The model under review builds one solid part; all positions refer to its coordinate system, in mm. Face numbers are marked on the shaded views. A direction names the side the tool comes from. Give positions to 0.01 mm unless a question says otherwise; leave off trailing zeros. Order: outer loops, then holes, each group sorted by start corner. A loop starts at its lowest first (then second) coordinate and runs counter-clockwise, first axis right, second up. Notation, with made-up numbers: (38.25, -13.5) - (73.25, -13.5) arc R15 ccw to (73.25, 10.5) - close; hole circle Ø9 at (-24, 30). An arc over 180 degrees is marked (long way). Use CSV: the item, a comma, the result in double quotes. Start each with the question number.
1. Take a section at D-D, the plane y = 19.5. State the section outline as (x, z) points.
2. Take a section at A-A, the plane z = 8.5. State the section outline as (x, y) points.
3. Machinability: for the marked faces 1, 2 and 3, which of the approach directions +Z, -Z, +X, -X, +Y, -Y give a long, thin tool a straight path to every point of the face, cutting with its end or side? Answer none if there is none.
4. Take a section at B-B, the plane x = -70.4. State the section outline as (y, z) points, then the cut area to 3 significant figures.
5. To check wall thickness, follow line 1 (Y direction, x = -70.4, z = 1); line 2 (X direction, y = 16.25, z = 16.75); line 3 (Z direction, x = -67.5, y = 13.5). State the ranges of each line that lie inside material, in increasing order. Write a range as [from, to].
6. For pin 1 (4 mm diameter, centred on x = -71, y = 17, fed in from +Z); pin 2 (2 mm diameter, centred on y = 25.38, z = 18.5, fed in from +X); pin 3 (3.5 mm diameter, centred on x = -83.5, z = 10.5, fed in from +Y), all flat-tipped, find the tip position at first contact; note any pin that passes through.
7. Take a section at C-C, the plane x = -75.75. State the section outline as (y, z) points.
```python
from build123d import *

# Parameters (mm, degrees)
SKETCH1_W                                 = 25
SKETCH1_H                                 = 20
BOSS_EXTRUDE1_DEPTH                       = 2
SKETCH2_W                                 = 2
SKETCH2_H                                 = 20
BOSS_EXTRUDE2_DEPTH                       = 23
FILLET2_R                                 = 1
FILLET3_R                                 = 1
RIB1_REACH                                = 94.888
SKETCH4_WALL_W                            = 204.746879862
SKETCH4_WALL_H                            = 2
CSK_FOR_0_FLAT_HEAD_MACHINE_SCREW_2_COUNT = 2
CSK_FOR_0_FLAT_HEAD_MACHINE_SCREW_2_PITCH = 10


with BuildPart() as part:
    # Sketch1 → Boss-Extrude1 (new body)
    with BuildSketch(Plane.XY):
        with Locations((-76.4, 19.882401427)):
            Rectangle(SKETCH1_W, SKETCH1_H)
    extrude(amount=BOSS_EXTRUDE1_DEPTH)

    # Sketch2 → Boss-Extrude2 (add)
    with BuildSketch(Plane.XY.offset(2)):
        with Locations((-87.9, 19.882401427)):
            Rectangle(SKETCH2_W, SKETCH2_H)
    extrude(amount=BOSS_EXTRUDE2_DEPTH)

    # Fillet2
    fillet2_edges = [part.edges().sort_by_distance(p)[0] for p in [
        (-86.9, 19.882401427, 2),
    ]]
    fillet(fillet2_edges, radius=FILLET2_R)

    # Fillet3
    fillet3_edges = [part.edges().sort_by_distance(p)[0] for p in [
        (-88.9, 19.882401427, 0),
    ]]
    fillet(fillet3_edges, radius=FILLET3_R)

    # Sketch4 wall → Rib1 (add, up to next)
    with BuildSketch(Plane(origin=(-80.9, 19.882401427, 8), x_dir=(0.707106781187, 0, -0.707106781187), z_dir=(0.707106781187, 0, 0.707106781187)), mode=Mode.PRIVATE) as rib1_sk1:
        Rectangle(SKETCH4_WALL_W, SKETCH4_WALL_H)
    rib1_tool1 = extrude(rib1_sk1.sketch, amount=-RIB1_REACH, mode=Mode.PRIVATE) - part.part
    add(rib1_tool1.solids().sort_by_distance((-80.9, 19.882401427, 8))[0])

    # Sketch5 → CSK for #0 Flat Head Machine Screw (100)1 (revolve, cut)
    with BuildSketch(Plane(origin=(-80.4, 14.382401427, 2), x_dir=(0, -1, 0), z_dir=(1, 0, 0))):
        Polygon((0, 0), (0, 10.53416509), (0.889, 10), (0.889, 0.5221717), (1.5113, 0), align=None)
    csk_for_0_flat_head_machine_screw_100 = revolve(axis=Axis((-80.4, 14.382401427, 8.35), (0, 0, -1)), mode=Mode.SUBTRACT)

    # CSK for _0 Flat Head Machine Screw _ 2: CSK for #0 Flat Head Machine Screw (100)1 ×2
    with Locations(*[(i * CSK_FOR_0_FLAT_HEAD_MACHINE_SCREW_2_PITCH, 0, 0) for i in range(1, CSK_FOR_0_FLAT_HEAD_MACHINE_SCREW_2_COUNT)]):
        add(csk_for_0_flat_head_machine_screw_100, mode=Mode.SUBTRACT)

    # Mirror1: CSK for #0 Flat Head Machine Screw (100)1 across plane
    add(csk_for_0_flat_head_machine_screw_100.mirror(Plane(origin=(0, 19.882401427, 0), x_dir=(0, 0, 1), z_dir=(0, -1, 0))), mode=Mode.SUBTRACT)

    # Mirror1 copy 1 sketch → Mirror1 copy 1 (revolve, cut)
    with BuildSketch(Plane(origin=(-70.4, 25.382401427, 2), x_dir=(0, 1, 0), z_dir=(1, 0, 0))):
        Polygon((0, 0), (0, -10.53416509), (0.889, -10), (0.889, -0.5221717), (1.5113, 0), align=None)
    revolve(axis=Axis((-70.4, 25.382401427, 8.35), (0, 0, 1)), mode=Mode.SUBTRACT)

    # Mirror2: CSK for #0 Flat Head Machine Screw (100)1 across plane
    add(csk_for_0_flat_head_machine_screw_100.mirror(Plane(origin=(-44.45, 0, 44.45), x_dir=(0.7071067811865481, 2.453269466693398e-15, 0.707106781186547), z_dir=(0.7071067811865471, 2.4532694666933947e-15, -0.707106781186548))), mode=Mode.SUBTRACT)

    # Mirror2 copy 1 sketch → Mirror2 copy 1 (revolve, cut)
    with BuildSketch(Plane(origin=(-86.9, 14.382401427, 18.5), x_dir=(0, -1, 0), z_dir=(0, 0, 1))):
        Polygon((0, 0), (0, -10.53416509), (0.889, -10), (0.889, -0.5221717), (1.5113, 0), align=None)
    revolve(axis=Axis((-80.55, 14.382401427, 18.5), (1, 0, 0)), mode=Mode.SUBTRACT)

    # Mirror2 copy 2 sketch → Mirror2 copy 2 (revolve, cut)
    with BuildSketch(Plane(origin=(-86.9, 25.382401427, 8.5), x_dir=(0, 1, 0), z_dir=(0, 0, 1))):
        Polygon((0, 0), (0, 10.53416509), (0.889, 10), (0.889, 0.5221717), (1.5113, 0), align=None)
    revolve(axis=Axis((-80.55, 25.382401427, 8.5), (-1, 0, 0)), mode=Mode.SUBTRACT)

    # Mirror2 copy 3 sketch → Mirror2 copy 3 (revolve, cut)
    with BuildSketch(Plane(origin=(-86.9, 25.382401427, 18.5), x_dir=(0, 1, 0), z_dir=(0, 0, 1))):
        Polygon((0, 0), (0, 10.53416509), (0.889, 10), (0.889, 0.5221717), (1.5113, 0), align=None)
    revolve(axis=Axis((-80.55, 25.382401427, 18.5), (-1, 0, 0)), mode=Mode.SUBTRACT)


solid = part.part
```
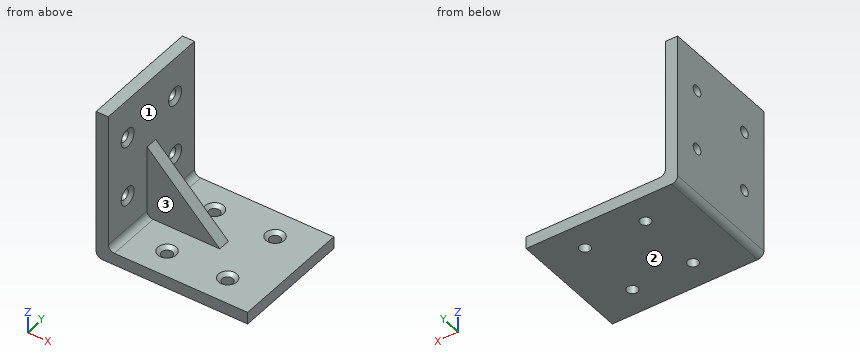
Determined:
1,outline,"(-88.9, 1) arc R1 ccw to (-87.9, 0) - (-63.9, 0) - (-63.9, 2) - (-74.9, 2) - (-86.9, 14) - (-86.9, 25) - (-88.9, 25) - close"
2,outline,"(-88.9, 9.88) - (-86.9, 9.88) - (-86.9, 12.87) - (-87.42, 13.49) - (-88.9, 13.49) - close; (-88.9, 15.27) - (-87.42, 15.27) - (-86.9, 15.89) - (-86.9, 18.88) - (-81.4, 18.88) - (-81.4, 20.88) - (-86.9, 20.88) - (-86.9, 23.87) - (-87.42, 24.49) - (-88.9, 24.49) - close; (-88.9, 26.27) - (-87.42, 26.27) - (-86.9, 26.89) - (-86.9, 29.88) - (-88.9, 29.88) - close"
3,face 1,"+Z, +X"
3,face 2,"-Z, +X, -X, +Y, -Y"
3,face 3,"+Z, +X, -Y"
4,outline,"(9.88, 0) - (13.49, 0) - (13.49, 1.48) - (12.87, 2) - (9.88, 2) - close; (15.27, 0) - (24.49, 0) - (24.49, 1.48) - (23.87, 2) - (15.89, 2) - (15.27, 1.48) - close; (26.27, 0) - (29.88, 0) - (29.88, 2) - (26.89, 2) - (26.27, 1.48) - close"
4,area,"32.2 mm²"
5,line 1,"y = [9.88, 13.49], [15.27, 24.49], [26.27, 29.88]"
5,line 2,"x = [-88.9, -86.9]"
5,line 3,"z = [0, 2]"
6,pin 1,"stops at z = 2"
6,pin 2,"stops at x = -87.33"
6,pin 3,"stops at y = 20.88"
7,outline,"(9.88, 0) - (29.88, 0) - (29.88, 2) - (20.88, 2) - (20.88, 2.85) - (18.88, 2.85) - (18.88, 2) - (9.88, 2) - close"
